Could you check a few things on this model? Use its own coordinates, in mm. A direction names the side the tool comes from. Give positions to 0.01 mm unless a question says otherwise; leave off trailing zeros. Order: outer loops, then holes, each group sorted by start corner. A loop starts at its lowest first (then second) coordinate and runs counter-clockwise, first axis right, second up. Notation, with made-up numbers: M 50.5,67.5 L 72.5,67.5 A12 ccw 72.5,87.5 Z; hole C 6,48.5 d11. An arc over 180 degrees is marked long. Answer in a Markdown table with one row per item. Add a question column.
```python
from build123d import *

# Parameters (mm, degrees)
F1_DEPTH = 10
F2_R     = 2
F3_DEPTH = 2
F4_R     = 4
F4_R_2   = 2
F5_DEPTH = 3
F6_R     = 1
F7_ANGLE = 90


# Not quite as in the source:
# - a feature names something its author has since deleted; it is built from what else it names


with BuildPart() as f1:
    # F0 (on Front) → F1 (new body, symmetric)
    with BuildSketch(Plane.XZ):
        Polygon((0, 5), (0, 0), (25, 0), (25, 1.3), (25, 5), align=None)
        Polygon((25, 0), (0, 0), (0, -5), (25, -5), (25, -1.3), align=None)
        Polygon((25, 5), (25, 1.3), (42, 1.3), (44, 1.3), (44, 5), align=None)
        Polygon((42, -1.3), (25, -1.3), (25, -5), (44, -5), (44, -1.3), align=None)
        Polygon((44, 1.3), (42, 1.3), (42, 0.75), align=None)
        Polygon((42, -0.75), (42, -1.3), (44, -1.3), align=None)
    extrude(amount=F1_DEPTH, both=True)

    # F2 (on face) → F3 (join)
    with BuildSketch(Plane(origin=(0, 0, 0), x_dir=(0, -1, 0), z_dir=(-1, 0, 0))):
        Circle(F2_R)
    extrude(amount=F3_DEPTH)

    # F4 (on face) → F5 (join)
    with BuildSketch(Plane(origin=(-2, 0, 0), x_dir=(0, -1, 0), z_dir=(-1, 0, 0))):
        Circle(F4_R)
        Circle(F4_R_2, mode=Mode.SUBTRACT)
        Circle(F4_R_2)
    extrude(amount=F5_DEPTH)

    # F6
    f6_edges = [f1.edges().sort_by_distance(p)[0] for p in [
        (44, -10, 3.15),
        (44, 10, 3.15),
        (44, 10, -3.15),
        (44, -10, -3.15),
        (0, -10, 0),
        (0, 10, 0),
        (0, 0, 5),
        (0, 0, -5),
        (44, 0, -5),
        (44, 0, 5),
        (33.5, -10, 1.3),
        (33.5, -10, -1.3),
        (25, -10, 0),
        (25, 10, 0),
        (33.5, 10, 1.3),
        (33.5, 10, -1.3),
    ]]
    fillet(f6_edges, radius=F6_R)


with BuildPart() as f1_1:
    # F7: moved
    add(f1.part.rotate(Axis((12.5, 0, 0), (1, 0, 0)), F7_ANGLE))


solid = f1_1.part
```
1. Will these pins go through, and if not, where does the flat tip stop? P1, Ø3, axis at y = 0, z = 3, coming from the +X side; P2, Ø4, axis at y = 3.5, z = 7.5, coming from the -X side.
2. If I drill on line 1 along X through (y, z) = (-1.5, -2); line 2 along Y through (x, z) = (32, -3.5); line 3 along X through (y, z) = (0.5, 3.5), over which ranges is the centre line in solid material (lowest first)? Write a range as [from, to].
3. Suppose I cut it at B-B on y = 0. List the corners of the cut face in (x, z) for me.
4. Thinking about a two-plate mould opening in X: for faces 1 (the cylindrical face through (0.285, 0.07, 9.699)), 2 (the flat face through (17, 0, -10)), 3 (the flat face through (33, -1.3, 0)), which applies, pulls with the +X half, pulls with the -X half, needs draft (parallel to the pull), parting line crosses it, or undercut?
5. For faces 4 (the cylindrical face through (24.6, 0, 9.8)), 5 (the flat face through (34, 1.3, 0)), 6 (the cylindrical face through (-3.479, 3.905, 0.867)), 7 (the cylindrical face through (-1, 2, 0)), 8 (the cylindrical face through (33.126, -1.601, -9.715)), which set-ups out of +Z, -Z, +X, -X, +Y, -Y let a thin tool reach every point of the face, with its end or its side?
6. Suppose I cut it at C-C on z = 0. List the corners of the cut face in (x, y) for me, plus the area to 3 significant figures.
7. Suppose I cut it at A-A on x = 27. List the corners of the cut face in (y, z) for me.
8. Suppose I cut it at D-D on y = -3.25. List the corners of the cut face in (x, z) for me, plus the area to 3 significant figures.
Findings below:
| question | item | result |
|---|---|---|
| 1 | P1 | x = 44 |
| 1 | P2 | x = 0 |
| 2 | line 1 | [-5, -2], [0, 44] |
| 2 | line 2 | [-5, -1.3], [1.3, 5] |
| 2 | line 3 | [-5, -2], [0, 25] |
| 3 | outline | M -5,-4 L -2,-4 L -2,-2 L 0,-2 L 0,-9 A1 ccw 1,-10 L 24,-10 A1 ccw 25,-9 L 25,9 A1 ccw 24,10 L 1,10 A1 ccw 0,9 L 0,2 L -2,2 L -2,4 L -5,4 Z |
| 4 | face 1 | pulls with the -X half |
| 4 | face 2 | needs draft |
| 4 | face 3 | undercut |
| 5 | face 4 | +Z |
| 5 | face 5 | +Z, -Z |
| 5 | face 6 | -X |
| 5 | face 7 | none |
| 5 | face 8 | -Z |
| 6 | outline | M -5,-4 L -2,-4 L -2,-2 L 0,-2 L 0,-4 A1 ccw 1,-5 L 43,-5 A1 ccw 44,-4 L 44,-1.3 L 42,-0.75 L 42,-1.3 L 25,-1.3 L 25,1.3 L 42,1.3 L 42,0.75 L 44,1.3 L 44,4 A1 ccw 43,5 L 1,5 A1 ccw 0,4 L 0,2 L -2,2 L -2,4 L -5,4 Z |
| 6 | area | 423 mm2 |
| 7 | outline | M -5,-10 L -2.3,-10 A1 ccw -1.3,-9 L -1.3,9 A1 ccw -2.3,10 L -5,10 Z; M 1.3,-9 A1 ccw 2.3,-10 L 5,-10 L 5,10 L 2.3,10 A1 ccw 1.3,9 Z |
| 8 | outline | M -5,-2.33 L -2,-2.33 L -2,2.33 L -5,2.33 Z; M 0,-9 A1 ccw 1,-10 L 43,-10 A1 ccw 44,-9 L 44,9 A1 ccw 43,10 L 1,10 A1 ccw 0,9 Z |
| 8 | area | 893 mm2 |
